The model under review builds one solid part; all positions refer to its coordinate system, in mm. A direction names the side the tool comes from. Round coordinates to 2 decimals unless told otherwise and drop trailing zeros. Write each loop counter-clockwise with the first axis right and the second up, starting at its lowest first coordinate (ties: lowest second). Pieces come first, ordered by that corner, then holes.
Item 1: Draft analysis for pull direction Z (two halves, no side actions). For faces 1 (the face through (-16, 25.4, 1)), 2 (the face through (-18.4, 18.2, -30.48)), 3 (the face through (-29.21, 13, -14)), 4 (the face through (-21.3, 12.5, 0)), state which applies: +Z half, -Z half, draft (parallel to the pull), parting line (faces both ways), or undercut.
Item 2: Add section B-B (z = -20). Give the boundary of the cut face in (x, y).
Item 3: Clearance check with a flat-ended pin moving along its axis: pin 1 Ø10 at (x, y) = (-18, 7.5) entering from -Z. State where the tip first meets the part, or that it passes through.
Item 4: Add section D-D (y = 4.75). Give the boundary of the cut face in (x, z), plus the area to 3 significant figures.
Item 5: Add section C-C (x = -27). Give the boundary of the cut face in (y, z).
Item 6: Machinability: for faces 5 (the face through (-19.285, 16.992, 0.644)), 6 (the face through (-21.3, 12.5, -29.21)), which of the approach directions +Z, -Z, +X, -X, +Y, -Y give a long, thin tool a straight path to every point of the face, cutting with its end or side? Answer none if there is none.
Item 7: To check wall thickness, follow L1, parallel to Z at x = -3.5, y = 11. State the ranges of the line that lie inside material, in increasing order.
Item 8: Add section A-A (y = 12.7). Give the boundary of the cut face in (x, z) (3 decimals), plus the area to 3 significant figures.
```python
from build123d import *

# Parameters (mm, degrees)
SKETCH1_W           = 31.75
SKETCH1_H           = 31.75
SKETCH1_W_2         = 29.21
SKETCH1_H_2         = 29.21
BOSS_EXTRUDE1_DEPTH = 25.4
CUT_EXTRUDE1_REACH  = 52.816
SKETCH2_R           = 6.35


with BuildPart() as part:
    # Sketch1 → Boss-Extrude1 (new body)
    with BuildSketch(Plane(origin=(0, 0, 0), x_dir=(1, 0, 0), z_dir=(0, 1, 0))):
        with Locations((-14.605, 14.605)):
            Rectangle(SKETCH1_W, SKETCH1_H)
        with Locations((-14.605, 14.605)):
            Rectangle(SKETCH1_W_2, SKETCH1_H_2, mode=Mode.SUBTRACT)
    extrude(amount=BOSS_EXTRUDE1_DEPTH)

    # Cut-Extrude1: up to this face of the body (flat: up to its plane)
    cut_extrude1_end = Plane(part.part.faces().sort_by_distance((-14.605, 12.7, -30.48))[0])
    # Sketch2 → Cut-Extrude1 (cut, up to the picked face)
    with BuildSketch(Plane.XY.offset(1.27), mode=Mode.PRIVATE) as cut_extrude1_sk1:
        with Locations((-14.605, 12.7)):
            Circle(SKETCH2_R)
    cut_extrude1_tool1 = split(extrude(cut_extrude1_sk1.sketch, amount=-CUT_EXTRUDE1_REACH, mode=Mode.PRIVATE), bisect_by=cut_extrude1_end, keep=Keep.BOTH, mode=Mode.PRIVATE)
    add(cut_extrude1_tool1.solids().sort_by(Axis((-14.605, 12.7, 1.27), (0, 0, -1)))[0], mode=Mode.SUBTRACT)


solid = part.part
```
Numbers:
1. face 1: draft
1. face 2: -Z half
1. face 3: undercut
1. face 4: undercut
2. outline: (-30.48, 0) - (-29.21, 0) - (-29.21, 25.4) - (-30.48, 25.4) - close; (0, 0) - (1.27, 0) - (1.27, 25.4) - (0, 25.4) - close
3. pin 1: stops at z = -30.48
4. outline: (-30.48, -30.48) - (1.27, -30.48) - (1.27, 1.27) - (-30.48, 1.27) - close; hole (-29.21, -29.21) - (0, -29.21) - (0, 0) - (-29.21, 0) - close
4. area: 155 mm2
5. outline: (0, -30.48) - (25.4, -30.48) - (25.4, -29.21) - (0, -29.21) - close; (0, 0) - (25.4, 0) - (25.4, 1.27) - (0, 1.27) - close
6. face 5: +Z, -Z
6. face 6: +Y, -Y
7. L1: z = -30.48 to -29.21, 0 to 1.27
8. outline: (-30.48, -30.48) - (-20.955, -30.48) - (-20.955, -29.21) - (-29.21, -29.21) - (-29.21, 0) - (-20.955, 0) - (-20.955, 1.27) - (-30.48, 1.27) - close; (-8.255, -30.48) - (1.27, -30.48) - (1.27, 1.27) - (-8.255, 1.27) - (-8.255, 0) - (0, 0) - (0, -29.21) - (-8.255, -29.21) - close
8. area: 123 mm2
